Model file for the job. Use its own axes, mm. A direction names the side the tool comes from. Give positions to 0.01 mm unless a question says otherwise; leave off trailing zeros. Order: outer loops, then holes, each group sorted by start corner. A loop starts at its lowest first (then second) coordinate and runs counter-clockwise, first axis right, second up. Notation, with made-up numbers: (-5.5, 50.5) - (37.5, 50.5) arc R20 ccw to (37.5, 60.5) - close; hole circle Ø7 at (78, 58.25). An arc over 180 degrees is marked (long way). Use CSV: the item, a comma, the result in double quotes. Start each with the question number.
(1) Band-saw the part on A-A, the plane x = 8. Give the cut face in (y, z).
(2) Pull direction Z, two halves, no side cores. Call faces 4 (the flat face through (50, 25, 25)), 5 (the flat face through (22, 25, 2)), 6 (the flat face through (46, 25, 25)), 7 (the flat face through (-1, 25, 52)): +Z half, -Z half, draft (parallel to the pull), parting line (faces both ways), or undercut.
(3) Tool access for faces 1 (the flat face through (25, 50, 25)), 2 (the flat face through (25, 25, 0)), 3 (the flat face through (22, 2, 25)): list every direction of +Z, -Z, +X, -X, +Y, -Y with a clear straight run to the whole face (end or side of a thin tool).
(4) Band-saw the part on B-B, the plane y = 9. Give the cut face in (x, z).
(5) Probe L1, parallel to Y at x = 37, z = 27; L2, parallel to X at y = 5.5, z = 31. List the from-to ranges inside material, lowest first.
(6) Drop flat-ended pins along their axis: pin 1 Ø5 at (x, z) = (27, 10.5) entering from +Y; pin 2 Ø1.5 at (y, z) = (10, 29) entering from -X; pin 3 Ø2 at (x, z) = (44.5, 28.5) entering from -Y. Give the stop position or say it passes through.
from build123d import *

# Parameters (mm, degrees)
BOX002_W     = 48
BOX002_H     = 46
BOX002_DEPTH = 46
BOX_W        = 50
BOX_H        = 50
BOX_DEPTH    = 50
BOX001_W     = 2
BOX001_H     = 54
BOX001_DEPTH = 54


with BuildPart() as cube002:
    # Box002 → Box002 (new body)
    with BuildSketch(Plane(origin=(-2, 2, 2), x_dir=(1, 0, 0), z_dir=(0, 0, 1))):
        with Locations((24, 23)):
            Rectangle(BOX002_W, BOX002_H)
    extrude(amount=BOX002_DEPTH)


with BuildPart() as cube:
    # Box → Box (new body)
    with BuildSketch(Plane.XY):
        with Locations((25, 25)):
            Rectangle(BOX_W, BOX_H)
    extrude(amount=BOX_DEPTH)


with BuildPart() as cut:
    # Box001 → Box001 (new body)
    with BuildSketch(Plane(origin=(-2, -2, -2), x_dir=(1, 0, 0), z_dir=(0, 0, 1))):
        with Locations((1, 27)):
            Rectangle(BOX001_W, BOX001_H)
    extrude(amount=BOX001_DEPTH)

    # Fusion: union Cube
    add(cube.part)

    # Cut: cut Cube002
    add(cube002.part, mode=Mode.SUBTRACT)


solid = cut.part
Answer block:
1,outline,"(0, 0) - (50, 0) - (50, 50) - (0, 50) - close; hole (2, 2) - (48, 2) - (48, 48) - (2, 48) - close"
2,face 4,"draft"
2,face 5,"undercut"
2,face 6,"undercut"
2,face 7,"+Z half"
3,face 1,"+Z, -Z, +X, +Y"
3,face 2,"-Z, +X, +Y, -Y"
3,face 3,"-X"
4,outline,"(-2, -2) - (0, -2) - (0, 0) - (50, 0) - (50, 50) - (0, 50) - (0, 52) - (-2, 52) - (-2, 48) - (46, 48) - (46, 2) - (-2, 2) - close"
5,L1,"y = 0 to 2, 48 to 50"
5,L2,"x = 46 to 50"
6,pin 1,"stops at y = 50"
6,pin 2,"stops at x = 46"
6,pin 3,"stops at y = 0"
